Geometry: final body of the model. Coordinates: model frame, mm. Face numbers are marked on the shaded views. A direction names the side the tool comes from. Give positions to 0.01 mm unless a question says otherwise; leave off trailing zeros. Write each loop counter-clockwise with the first axis right and the second up, starting at its lowest first coordinate (ties: lowest second). Pieces come first, ordered by that corner, then holes. Notation, with made-up numbers: (-39.5, 70) -> (-32.5, 70) arc R34 ccw to (-32.5, 106) -> close; hole circle Ø5 at (46.5, -34). An arc over 180 degrees is marked (long way). Answer in a Markdown table with one row per item. Add a question column.
Item 1: Section query A-A on x = 10. Output: boundary loops of the cut face in (y, z).
Item 2: Section query C-C on z = 0.75. Output: boundary loops of the cut face in (x, y), plus the area to 3 significant figures.
Item 3: Draft query along Y for the marked faces 1, 2 and 3. Return one class per face: +Y half, -Y half, draft (parallel to the pull), parting line (faces both ways), or undercut.
Item 4: Section query B-B on y = 6.5. Output: boundary loops of the cut face in (x, z), plus the area to 3 significant figures.
Item 5: First-contact query: P1, Ø4, axis at x = 21.5, y = 3, coming from the +Z side; P2, Ø1.5, axis at x = 11, z = 1.5, coming from the -Y side; P3, Ø2, axis at x = 1.88, y = 3.91, coming from the -Z side; P4, Ø0.9, axis at x = 6, z = 1, coming from the +Y side. Flat tips, straight axial feed; report the tip coordinate or a pass-through.
Item 6: Access query for the marked faces 4, 5, 6 and 7. Directions: +Z, -Z, +X, -X, +Y, -Y. A direction counts if a zero-diameter tool reaches every point of the face in a straight line with its end or side. Return the directions, or none.
Item 7: Material intervals for probe 1 along Y at (x, z) = (9.5, 1.6); probe 2 along X at (y, z) = (4.75, 1); probe 3 along X at (y, z) = (6, 2.1), sorted ascending. Write a range as from..to.
Item 8: Section query D-D on y = 3.25. Output: boundary loops of the cut face in (x, z).
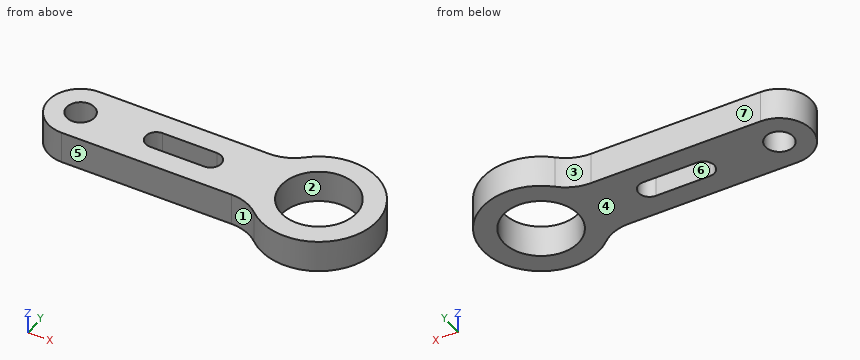
```python
from build123d import *

# Parameters (mm, degrees)
SKETCH_1_R      = 3.5
SKETCH_1_R_2    = 1.3
EXTRUDE_1_DEPTH = 3


with BuildPart() as part:
    # 草图1 → 凸台-拉伸1 (new body)
    with BuildSketch(Plane.XY.offset(3)):
        with BuildLine():
            Line((17.542771769, 6.907119873), (1.879793686, 6.907119873))
            ThreePointArc((1.879793686, 6.907119873), (-1.120206314, 3.907119873), (1.879793686, 0.907119873))
            Line((1.879793686, 0.907119873), (17.544137719, 0.907119873))
            ThreePointArc((17.544137719, 0.907119873), (18.981359081, 0.640000095), (20.226625317, -0.125682749))
            ThreePointArc((20.226625317, -0.125682749), (29.310375688, 3.908267946), (20.225838323, 7.940446))
            ThreePointArc((20.225838323, 7.940446), (18.980357333, 7.174379894), (17.542771769, 6.907119873))
        make_face()
        with Locations(Location((23.87302906, 3.907737435, 0), (0, 0, 180))):
            Circle(SKETCH_1_R, mode=Mode.SUBTRACT)
        with Locations(Location((1.88402906, 3.907119873, 0), (0, 0, 180))):
            Circle(SKETCH_1_R_2, mode=Mode.SUBTRACT)
        with BuildLine():
            Line((8.87402906, 4.907386497), (13.87402906, 4.907386497))
            ThreePointArc((13.87402906, 4.907386497), (14.87402906, 3.907386497), (13.87402906, 2.907386497))
            Line((13.87402906, 2.907386497), (8.87402906, 2.907386497))
            ThreePointArc((8.87402906, 2.907386497), (7.87402906, 3.907386497), (8.87402906, 4.907386497))
        make_face(mode=Mode.SUBTRACT)
    extrude(amount=-EXTRUDE_1_DEPTH)


solid = part.part
```
Findings below:
| question | item | result |
|---|---|---|
| 1 | outline | (0.91, 0) -> (2.91, 0) -> (2.91, 3) -> (0.91, 3) -> close; (4.91, 0) -> (6.91, 0) -> (6.91, 3) -> (4.91, 3) -> close |
| 2 | outline | (1.88, 0.91) -> (17.54, 0.91) arc R4 cw to (20.23, -0.13) arc R5.44 ccw (long way) to (20.23, 7.94) arc R4 cw to (17.54, 6.91) -> (1.88, 6.91) arc R3 ccw to start; hole circle Ø2.6 at (1.88, 3.91); hole (8.87, 2.91) -> (13.87, 2.91) arc R1 ccw to (13.87, 4.91) -> (8.87, 4.91) arc R1 ccw to start; hole circle Ø7 at (23.87, 3.91) |
| 2 | area | 152 mm^2 |
| 3 | face 1 | -Y half |
| 3 | face 2 | undercut |
| 3 | face 3 | +Y half |
| 4 | outline | (0.37, 0) -> (21.52, 0) -> (21.52, 3) -> (0.37, 3) -> close; (26.22, 0) -> (28.65, 0) -> (28.65, 3) -> (26.22, 3) -> close |
| 4 | area | 70.7 mm^2 |
| 5 | P1 | stops at z = 3 |
| 5 | P2 | stops at y = 0.91 |
| 5 | P3 | passes through |
| 5 | P4 | stops at y = 6.91 |
| 6 | face 4 | -Z, +X, -X, +Y, -Y |
| 6 | face 5 | +Z, -Z, -X, -Y |
| 6 | face 6 | +Z, -Z |
| 6 | face 7 | +Z, -Z, -X, +Y |
| 7 | probe 1 | y = 0.91..2.91, 4.91..6.91 |
| 7 | probe 2 | x = -1..0.89, 2.87..8.34, 14.41..20.48, 27.27..29.24 |
| 7 | probe 3 | x = -0.27..21.07, 26.68..28.89 |
| 8 | outline | (-1.05, 0) -> (0.76, 0) -> (0.76, 3) -> (-1.05, 3) -> close; (3.01, 0) -> (8.12, 0) -> (8.12, 3) -> (3.01, 3) -> close; (14.63, 0) -> (20.44, 0) -> (20.44, 3) -> (14.63, 3) -> close; (27.31, 0) -> (29.27, 0) -> (29.27, 3) -> (27.31, 3) -> close |
